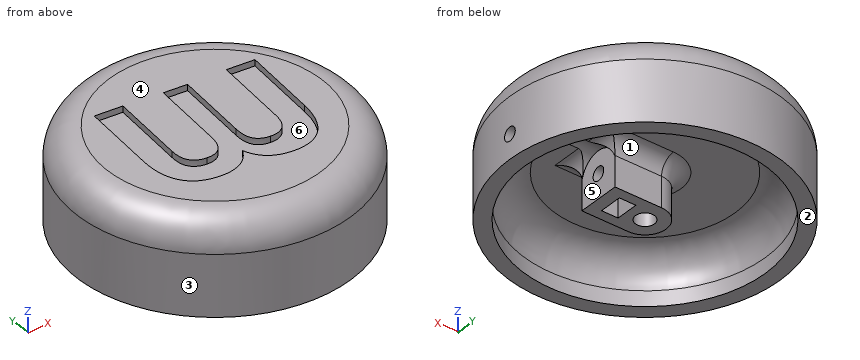
```python
from build123d import *

# Parameters (mm, degrees)
ESQUISSE1_R                  = 45
BOSS_EXTRU_1_DEPTH           = 30
CONG_1_R                     = 10
ESQUISSE3_R                  = 40
ESQUISSE3_R_2                = 7
ESQUISSE3_R_3                = 3.15
ENL_V_MAT_EXTRU_1_DEPTH      = 15
CONG_2_R                     = 10
ENL_V_MAT_EXTRU_2_DEPTH      = 2
BOSS_EXTRU_3_DEPTH           = 22
ENL_V_MAT_EXTRU_3_DEPTH      = 8
ESQUISSE14_W                 = 8
ESQUISSE14_H                 = 7.5
ENL_V_MAT_EXTRU_4_DEPTH      = 8
ESQUISSE15_W                 = 1.5
ESQUISSE15_H                 = 14
ESQUISSE15_W_2               = 2.5
BOSS_EXTRU_4_DEPTH           = 15
ENL_V_MAT_EXTRU_5_DEPTH      = 31
ENL_V_MAT_EXTRU_5_DEPTH_BACK = 15
ESQUISSE16_R                 = 2.25
CONG_3_R                     = 5
ESQUISSE17_R                 = 7
ENL_V_MAT_EXTRU_6_DEPTH      = 8


with BuildPart() as part:
    # Esquisse1 → Boss.-Extru.1 (new body)
    with BuildSketch(Plane.XY):
        Circle(ESQUISSE1_R)
    extrude(amount=BOSS_EXTRU_1_DEPTH)

    # Congé1
    cong_1_edges = [part.edges().sort_by_distance(p)[0] for p in [
        (-45, 0, 30),
    ]]
    fillet(cong_1_edges, radius=CONG_1_R)

    # Esquisse3 → Enlèv. mat.-Extru.1 (cut)
    # profile 1 of 2: a face of its own
    with BuildSketch(Plane(origin=(0, 0, 0), x_dir=(-1, 0, 0), z_dir=(0, 0, -1))):
        Circle(ESQUISSE3_R)
        Circle(ESQUISSE3_R_2, mode=Mode.SUBTRACT)
    # profile 2 of 2: a face of its own
    with BuildSketch(Plane(origin=(0, 0, 0), x_dir=(-1, 0, 0), z_dir=(0, 0, -1))):
        Circle(ESQUISSE3_R_3)
    extrude(amount=-ENL_V_MAT_EXTRU_1_DEPTH, mode=Mode.SUBTRACT)

    # Congé2
    cong_2_edges = [part.edges().sort_by_distance(p)[0] for p in [
        (40, 0, 15),
    ]]
    fillet(cong_2_edges, radius=CONG_2_R)

    # Esquisse4 → Enlèv. mat.-Extru.2 (cut)
    with BuildSketch(Plane.XY.offset(30)):
        with BuildLine():
            Line((-22.144645679, 22.871728166), (-13.411684949, 21.864078851))
            Line((-13.411684949, 21.864078851), (-16.224705953, -2.434964528))
            add(Edge.make_bspline(
                [(-16.224705953, -2.434964528), (-16.256895394, -2.749529996), (-16.318662647, -3.353139284), (-16.340974486, -4.233864403), (-16.297568174, -5.05080651), (-16.209258973, -5.810700887), (-16.049709468, -6.510266382), (-15.835926627, -7.151237119), (-15.544352246, -7.724871201), (-15.102471016, -8.410829584), (-14.391447141, -9.137358845), (-13.364077291, -9.804334199), (-12.168771745, -10.281809796), (-11.302704519, -10.415743134), (-10.850576273, -10.485662702)],
                knots=[0, 0, 0, 0, 1.029052784, 1.9746154, 2.864125884, 3.690516433, 4.461360084, 5.196106019, 5.883704519, 6.550229516, 7.847027763, 9.154782256, 10.514661136, 12, 12, 12, 12], degree=3))
            add(Edge.make_bspline(
                [(-10.850576273, -10.485662702), (-10.388538715, -10.518722359), (-9.507769114, -10.581743082), (-8.241462414, -10.373028261), (-7.130743608, -9.898839405), (-6.180259361, -9.165116879), (-5.41633373, -8.159424838), (-4.807311446, -6.915829185), (-4.36244309, -5.421735756), (-4.205585893, -4.334155707), (-4.122417825, -3.757504254)],
                knots=[0, 0, 0, 0, 1.021408317, 1.94708283, 2.80626198, 3.666415336, 4.56998295, 5.573071206, 6.71320551, 8, 8, 8, 8], degree=3))
            Line((-4.122417825, -3.757504254), (-1.361878556, 20.100692549))
            Line((-1.361878556, 20.100692549), (6.027549754, 19.239992093))
            Line((6.027549754, 19.239992093), (3.246017791, -4.838627999))
            add(Edge.make_bspline(
                [(3.246017791, -4.838627999), (3.195337805, -5.418932779), (3.100060271, -6.509896153), (3.200846418, -8.063631191), (3.502191789, -9.416150043), (4.030577709, -10.569421741), (4.79817358, -11.502650362), (5.789145136, -12.206937692), (6.981097787, -12.714787486), (7.862811963, -12.849833616), (8.326249754, -12.920815213)],
                knots=[0, 0, 0, 0, 1.281245697, 2.408720684, 3.414105471, 4.317064152, 5.176266696, 6.042350125, 6.971039643, 8, 8, 8, 8], degree=3))
            add(Edge.make_bspline(
                [(8.326249754, -12.920815213), (8.788141435, -12.95187261), (9.670978885, -13.011234217), (10.951767235, -12.825942037), (12.09662951, -12.373936159), (12.926595681, -11.793896672), (13.517779888, -11.226565316), (13.904051152, -10.714814626), (14.251276342, -10.139874431), (14.570575393, -9.505698745), (14.812975228, -8.791702106), (15.036199887, -8.026114103), (15.218288171, -7.192139962), (15.290111141, -6.609767539), (15.327313225, -6.308116583)],
                knots=[0, 0, 0, 0, 1.514963289, 2.895627662, 4.203605979, 5.514649424, 6.187972473, 6.883219808, 7.609208956, 8.389033415, 9.205462736, 10.07686117, 11.003873391, 12, 12, 12, 12], degree=3))
            Line((15.327313225, -6.308116583), (18.17182327, 18.274328166))
            Line((18.17182327, 18.274328166), (26.904784001, 17.266678851))
            Line((26.904784001, 17.266678851), (24.060273955, -7.315765898))
            add(Edge.make_bspline(
                [(24.060273955, -7.315765898), (23.967955783, -8.006475678), (23.789795838, -9.339439852), (23.384357503, -11.243708182), (22.85722021, -12.976937412), (22.232797618, -14.545925787), (21.501446812, -15.949427752), (20.701837208, -17.210493748), (19.823941524, -18.330780706), (18.850170073, -19.291918516), (17.80713126, -20.105941628), (16.692463853, -20.773870797), (15.510213899, -21.304477515), (14.25612176, -21.680062816), (12.955241569, -21.910077191), (11.619045856, -22.055429721), (10.247905107, -22.064471081), (9.32643267, -21.979861564), (8.861563453, -21.937177314)],
                knots=[0, 0, 0, 0, 1.394876439, 2.691898066, 3.892940253, 5.018147218, 6.067743577, 7.056852335, 8.004277114, 8.910753966, 9.789328284, 10.647102319, 11.506305359, 12.377222316, 13.26067029, 14.147997917, 15.065692338, 16, 16, 16, 16], degree=3))
            add(Edge.make_bspline(
                [(8.861563453, -21.937177314), (8.193397296, -21.838611708), (6.905963094, -21.64869378), (5.09075363, -21.099474321), (3.476356998, -20.341045448), (2.056804317, -19.378476271), (0.854405876, -18.205860501), (-0.171754699, -16.868311251), (-0.984609243, -15.338236734), (-1.366188524, -14.231821472), (-1.56130915, -13.666055852)],
                knots=[0, 0, 0, 0, 1.141163769, 2.198814248, 3.194086385, 4.147709345, 5.085148259, 6.022512461, 6.988811434, 8, 8, 8, 8], degree=3))
            add(Edge.make_bspline(
                [(-1.56130915, -13.666055852), (-1.871640737, -14.180350205), (-2.475746289, -15.181498932), (-3.614218819, -16.476909983), (-4.899960101, -17.530118409), (-6.330522074, -18.355291156), (-7.908683346, -18.929201697), (-9.627036508, -19.274410878), (-11.485566119, -19.393346682), (-12.761481825, -19.278232362), (-13.422181296, -19.218623432)],
                knots=[0, 0, 0, 0, 1.028409916, 2.001949416, 2.939882333, 3.867066551, 4.819923276, 5.805897814, 6.863841753, 8, 8, 8, 8], degree=3))
            add(Edge.make_bspline(
                [(-13.422181296, -19.218623432), (-13.899737749, -19.154485913), (-14.838533125, -19.028402376), (-16.198819588, -18.681486488), (-17.495358388, -18.246704571), (-18.716659117, -17.688648624), (-19.854452529, -17.019622786), (-20.894753111, -16.223737722), (-21.831175407, -15.306627023), (-22.667865015, -14.26853153), (-23.394554113, -13.106606892), (-24.004820997, -11.821339515), (-24.481775919, -10.4096633), (-24.866331461, -8.881644272), (-25.105076103, -7.214751414), (-25.186086506, -5.41002077), (-25.163088385, -3.462876846), (-25.027862816, -2.122901673), (-24.957666684, -1.427315213)],
                knots=[0, 0, 0, 0, 0.95812083, 1.883503822, 2.788440276, 3.676396848, 4.550459974, 5.409672077, 6.276215641, 7.152632684, 8.056711632, 8.997240929, 9.97707405, 11.017285228, 12.128953384, 13.32118734, 14.609417657, 16, 16, 16, 16], degree=3))
            Line((-24.957666684, -1.427315213), (-22.144645679, 22.871728166))
        make_face()
    extrude(amount=-ENL_V_MAT_EXTRU_2_DEPTH, mode=Mode.SUBTRACT)

    # Esquisse12 → Boss.-Extru.3 (add)
    with BuildSketch(Plane(origin=(0, 0, 0), x_dir=(-1, 0, 0), z_dir=(0, 0, -1))):
        with BuildLine():
            ThreePointArc((0, 7), (-7, 0), (0, -7))
            Line((0, -7), (0, -3.15))
            ThreePointArc((0, -3.15), (-3.15, 0), (0, 3.15))
            Line((0, 3.15), (0, 7))
        make_face()
        with BuildLine():
            Line((0, -3.15), (0, -7))
            ThreePointArc((0, -7), (4.949747468, -4.949747468), (7, 0))
            ThreePointArc((7, 0), (4.949747468, 4.949747468), (0, 7))
            Line((0, 7), (0, 3.15))
            ThreePointArc((0, 3.15), (2.227386361, 2.227386361), (3.15, 0))
            ThreePointArc((3.15, 0), (2.227386361, -2.227386361), (0, -3.15))
        make_face()
        with BuildLine():
            Line((-14, -7), (0, -7))
            ThreePointArc((0, -7), (-7, 0), (0, 7))
            Line((0, 7), (-14, 7))
            Line((-14, 7), (-14, -7))
        make_face()
    extrude(amount=-BOSS_EXTRU_3_DEPTH)

    # Esquisse13 → Enlèv. mat.-Extru.3 (cut)
    with BuildSketch(Plane(origin=(14, 0, 0), x_dir=(0, 0, -1), z_dir=(1, 0, 0))):
        Polygon((-10.165063509, 3.75), (-12.330127019, 0), (-10.165063509, -3.75), (-5.834936491, -3.75), (-3.669872981, 0), (-5.834936491, 3.75), align=None)
    extrude(amount=-ENL_V_MAT_EXTRU_3_DEPTH, mode=Mode.SUBTRACT)

    # Esquisse14 → Enlèv. mat.-Extru.4 (cut)
    with BuildSketch(Plane(origin=(0, 0, 0), x_dir=(-1, 0, 0), z_dir=(0, 0, -1))):
        with Locations((-10, 0)):
            Rectangle(ESQUISSE14_W, ESQUISSE14_H)
    extrude(amount=-ENL_V_MAT_EXTRU_4_DEPTH, mode=Mode.SUBTRACT)

    # Esquisse15 → Boss.-Extru.4 (add)
    with BuildSketch(Plane(origin=(0, 0, 15), x_dir=(-1, 0, 0), z_dir=(0, 0, -1))):
        with Locations((-14.75, 0)):
            Rectangle(ESQUISSE15_W, ESQUISSE15_H)
        with Locations((-12.75, 0)):
            Rectangle(ESQUISSE15_W_2, ESQUISSE15_H)
    extrude(amount=BOSS_EXTRU_4_DEPTH)

    # Esquisse16 → Enlèv. mat.-Extru.5 (cut, two sides: drawn at the far end of the back side and taken through both)
    with BuildSketch(Plane(origin=(15.5, 0, 0), x_dir=(0, 0, -1), z_dir=(1, 0, 0)).offset(-ENL_V_MAT_EXTRU_5_DEPTH_BACK)):
        with Locations(Location((-8, 0, 0), (0, 0, 180))):
            Circle(ESQUISSE16_R)
    extrude(amount=ENL_V_MAT_EXTRU_5_DEPTH + ENL_V_MAT_EXTRU_5_DEPTH_BACK, mode=Mode.SUBTRACT)

    # Congé3
    cong_3_edges = [part.edges().sort_by_distance(p)[0] for p in [
        (15.5, 0, 15),
        (-7, 0, 15),
        (7.75, -7, 15),
        (7.75, 7, 15),
    ]]
    fillet(cong_3_edges, radius=CONG_3_R)

    # Esquisse17 → Enlèv. mat.-Extru.6 (cut)
    with BuildSketch(Plane(origin=(15.5, 0, 0), x_dir=(0, 0, -1), z_dir=(1, 0, 0))):
        with Locations((-8.317654901, 0)):
            Circle(ESQUISSE17_R)
    extrude(amount=ENL_V_MAT_EXTRU_6_DEPTH, mode=Mode.SUBTRACT)


solid = part.part
```
Here's how the part is built. I have some questions about the finished solid (model axes, mm). Face numbers are marked on the shaded views. A direction names the side the tool comes from. Give positions to 0.01 mm unless a question says otherwise; leave off trailing zeros. Write each loop counter-clockwise with the first axis right and the second up, starting at its lowest first coordinate (ties: lowest second). Pieces come first, ordered by that corner, then holes.
(1) On a 3-axis mill with a long thin cutter (end or side, diameter ignored), from which of +Z, -Z, +X, -X, +Y, -Y can I reach the whole of each face in a straight line? I mean the marked faces 4, 5 and 6. Say none if no direction works.
Output values:
face 4: +Z, +X, -X, +Y, -Y
face 5: -Z
face 6: +Z
(2) Imagine slicing it at C-C, the plane z = 24. Write out the boundary of the cut face in (x, y), and give its area (3 significant figures).
Output values:
outline: circle Ø88.33 at (0, 0)
area: 6,130 mm2
(3) If I drill on L1, parallel to Y at x = 0, z = 1; L2, parallel to Y at x = 4, z = 8; L3, parallel to X at y = 5, z = 12.5, over which ranges is the centre line in solid material (lowest first)?
Output values:
L1: y = -45 to -40, -7 to -3.15, 3.15 to 7, 40 to 45
L2: y = -44.82 to -39.34, -7 to -2.25, 2.25 to 7, 39.34 to 44.82
L3: x = -44.72 to -36.27, -5.82 to 15.5, 36.27 to 44.72
(4) Thinking about a two-plate mould opening in Y: for the marked faces 1, 2 and 3, which applies, pulls with the +Y half, pulls with the -Y half, needs draft (parallel to the pull), parting line crosses it, or undercut?
Output values:
face 1: undercut
face 2: needs draft
face 3: parting line crosses it
(5) Imagine slicing it at A-A, the plane z = 3. Write out the boundary of the cut face in (x, y), and give its area (3 significant figures).
Output values:
outline: circle Ø90 at (0, 0); (0, -7) - (15.5, -7) - (15.5, 7) - (0, 7) arc R7 ccw to start; hole circle Ø80 at (0, 0); hole circle Ø6.3 at (0, 0); hole (6, -3.75) - (11.5, -3.75) - (11.5, 3.75) - (6, 3.75) - close
area: 1,560 mm2
(6) Imagine slicing it at B-B, the plane z = 8. Write out the boundary of the cut face in (x, y).
Output values:
outline: (0, -7) - (15.5, -7) - (15.5, -2.25) - (11.5, -2.25) - (11.5, -3.75) - (6, -3.75) - (6, -2.25) - (2.2, -2.25) arc R3.15 cw (long way) to (2.2, 2.25) - (6, 2.25) - (6, 3.75) - (11.5, 3.75) - (11.5, 2.25) - (15.5, 2.25) - (15.5, 7) - (0, 7) arc R7 ccw to start; (39.48, -2.25) arc R39.54 cw (long way) to (39.48, 2.25) - (44.94, 2.25) arc R45 ccw (long way) to (44.94, -2.25) - close
(7) Will these pins go through, and if not, where does the flat tip stop? pin 1 (2 mm diameter, centred on x = -21.5, z = 19, fed in from +Y); pin 2 (8 mm diameter, centred on x = -21, z = 5, fed in from +Y); pin 3 (1 mm diameter, centred on y = -19.5, z = 15.5, fed in from +X).
Output values:
pin 1: stops at y = 40.06
pin 2: stops at y = 41.67
pin 3: stops at x = 40.79
